The model under review builds one solid part; all positions refer to its coordinate system, in mm. Face numbers are marked on the shaded views. A direction names the side the tool comes from. Round coordinates to 2 decimals unless told otherwise and drop trailing zeros. Loops run counter-clockwise (first coordinate to the right, second up) from the corner with the lowest first, then second, coordinate; pieces in that order, holes last. Notation, with made-up numbers: M 78.25,-16.5 L 85.25,-16.5 A17 cw 85.25,9.5 Z; hole C 56,3.25 d11. An arc over 180 degrees is marked long. Answer as a JSON object with one key per item and string values. Group by question number.
Item 1: Insertion check: P1, Ø1.6, axis at x = -70, z = -13.5, coming from the -Y side; P2, Ø3, axis at x = 154, y = -99, coming from the -Z side; P3, Ø1, axis at y = -211.5, z = -12.5, coming from the -X side. Each pin has a flat end and moves straight along its axis. Give the tip position at first contact, or say it passes through.
Item 2: Consider section A-A (y = -86). Give the boundary of the cut face in (x, z) (3 decimals), and give its area (3 significant figures).
Item 3: Consider section D-D (y = -206). Give the boundary of the cut face in (x, z) (3 decimals), and give its area (3 significant figures).
Item 4: Consider section B-B (x = -65.5). Give the boundary of the cut face in (y, z).
Item 5: Consider section C-C (z = 36.5). Give the boundary of the cut face in (x, y), and give its area (3 significant figures).
Item 6: To check wall thickness, follow line 1 (Z direction, x = 13.5, y = -63); line 2 (X direction, y = -210.5, z = 61); line 3 (X direction, y = -215.5, z = 3.5). State the ranges of each line that lie inside material, in increasing order.
Item 7: Tool access review of the marked faces 1 and 2: name each direction out of +Z, -Z, +X, -X, +Y, -Y from which nothing blocks a thin tool from reaching the whole face with its end or side.
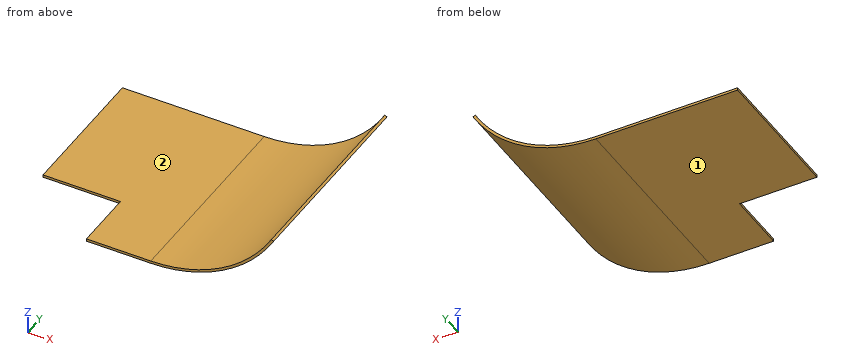
```python
from build123d import *

# Parameters (mm, degrees)
F1_DEPTH = 177.8
F3_DEPTH = 76.2


with BuildPart() as f1:
    # F0 (on Front) → F1 (new body)
    with BuildSketch(Plane.XZ):
        with BuildLine():
            Line((-97.126943, -11.306872), (-97.126943, -14.481872))
            Line((-97.126943, -14.481872), (80.673057, -14.481872))
            ThreePointArc((80.673057, -14.481872), (169.573057, 9.338811), (234.652374, 74.418128))
            Line((234.652374, 74.418128), (231.902743, 76.005628))
            ThreePointArc((231.902743, 76.005628), (167.985557, 12.088441), (80.673057, -11.306872))
            Line((80.673057, -11.306872), (-97.126943, -11.306872))
        make_face()
    extrude(amount=F1_DEPTH)

    # F2 (on face) → F3 (join)
    with BuildSketch(Plane.XZ.offset(177.8)):
        with BuildLine():
            Line((80.673057, -11.306872), (0, -11.306872))
            Line((0, -11.306872), (0, -14.481872))
            Line((0, -14.481872), (25.070544, -14.481872))
            Line((25.070544, -14.481872), (80.673057, -14.481872))
            ThreePointArc((80.673057, -14.481872), (169.573057, 9.338811), (234.652374, 74.418128))
            Line((234.652374, 74.418128), (231.902743, 76.005628))
            ThreePointArc((231.902743, 76.005628), (167.985557, 12.088441), (80.673057, -11.306872))
        make_face()
    extrude(amount=F3_DEPTH)


solid = f1.part
```
Geometry results:
{
 "1": {"P1": "stops at y = -177.8", "P2": "stops at z = 0.67", "P3": "stops at x = 0"},
 "2": {"outline": "M -97.127,-14.482 L 80.673,-14.482 A177.8 ccw 234.652,74.418 L 231.903,76.006 A174.625 cw 80.673,-11.307 L -97.127,-11.307 Z", "area": "1,150 mm^2"},
 "3": {"outline": "M 0,-14.482 L 80.673,-14.482 A177.8 ccw 234.652,74.418 L 231.903,76.006 A174.625 cw 80.673,-11.307 L 0,-11.307 Z", "area": "842 mm^2"},
 "4": {"outline": "M -177.8,-14.48 L 0,-14.48 L 0,-11.31 L -177.8,-11.31 Z"},
 "5": {"outline": "M 200.72,-254 L 205.29,-254 L 205.29,0 L 200.72,0 Z", "area": "1,160 mm^2"},
 "6": {"line 1": "z = -14.48 to -11.31", "line 2": "x = 222.18 to 226.08", "line 3": "x = 151.04 to 158.59"},
 "7": {"face 1": "-Z, +X, -X, +Y, -Y", "face 2": "+Z, -X, +Y, -Y"}
}
